Autodesk Inventor part; units mm, degrees
ref_plane "YZ Plane" through (0, 0, 0) normal (1, 0, 0) x (0, 1, 0)
ref_plane "XZ Plane" through (0, 0, 0) normal (0, 1, 0) x (-1, 0, 0)
ref_plane "XY Plane" through (0, 0, 0) normal (0, 0, 1) x (1, 0, 0)
sketch "Sketch1" plane through (0, 0, 0) normal (1, 0, 0) x (0, 1, 0)
  line L0 (50, 50) -> (-50, 50)
  line L1 (-50, 50) -> (-50, -50)
  line L2 (-50, -50) -> (50, -50)
  line L3 (50, -50) -> (50, 50)
  line L4 (50, 50) -> (-50, -50) construction
  line L5 (-50, 50) -> (50, -50) construction
  point P0 (0, 0)
  dimension "d0" = 100
  dimension "d1" = 100
extrude "Extrusion1" add sketch "Sketch1" along normal blind 3
sketch "Sketch2" plane through (3, 0, 0) normal (1, 0, 0) x (0, 0, -1)
  circle A0 centre (-8, -9) radius 1.5
  circle A1 centre (8, -9) radius 1.5
  circle A2 centre (8, 9) radius 1.5
  circle A3 centre (-8, 9) radius 1.5
  ellipse E0 centre (0, 0) end of major axis (13, 14) minor radius 3.6924 (4.9841, 0.0284) -> (0.0262, 5.3386) ccw
  ellipse E1 centre (0, 0) end of major axis (-13, 14) minor radius 3.7302 (0.0262, 5.3386) -> (-4.9841, -0.0284) ccw
  ellipse E2 centre (0, 0) end of major axis (13, 14) minor radius 3.6924 (-4.9841, -0.0284) -> (-0.0262, -5.3386) ccw
  ellipse E3 centre (0, 0) end of major axis (-13, 14) minor radius 3.7302 (-0.0262, -5.3386) -> (4.9841, 0.0284) ccw
  point P0 (0, 9.3923)
extrude "Extrusion2" cut sketch "Sketch2" against normal blind 3 contours A0 | A1 | A2 | A3
sketch "Sketch3" plane through (3, 0, 0) normal (1, 0, 0) x (0, 0, -1)
  circle A0 centre (0, 0) radius 2.2245
extrude "Extrusion3" cut sketch "Sketch3" against normal blind 1
properties part number "marker plate"
Input: part model. Units: mm. Frame: model coordinates. A direction names the side the tool comes from. Coordinates: 2 decimals unless noted, no trailing zeros. Loops run counter-clockwise (first coordinate to the right, second up) from the corner with the lowest first, then second, coordinate; pieces in that order, holes last. Notation, with made-up numbers: (-17.75, 44.5) - (26.25, 44.5) arc R21 cw to (26.25, 73.5) - close; hole circle Ø10 at (28, 89.5). An arc over 180 degrees is marked (long way). Answer in a Markdown table with one row per item. Add a question column.
Item 1: Section query A-A on y = -9. Return the cut outline in (x, z), then the cut area to 3 significant figures.
Item 2: Section query B-B on z = 8. Return the cut outline in (x, y).
Item 3: Line query: line 1 along Y through (x, z) = (1.05, 8); line 2 along Y through (x, z) = (2.55, 0); line 3 along Z through (x, y) = (2.7, -0.5). Output: solid intervals per line, ascending. Write a range as [from, to].
Item 4: Access query for faces 1 (the flat face through (3, -1, 12)), 2 (the cylindrical face through (2.51, 0.67, -2.12)). Directions: +Z, -Z, +X, -X, +Y, -Y. A direction counts if a zero-diameter tool reaches every point of the face in a straight line with its end or side. Return the directions, or none.
Item 5: Mould query, pull axis Y, two halves, no side actions, for faces 3 (the cylindrical face through (1.5, -9.9, 9.2)), 4 (the flat face through (1, 50, -1)), 5 (the flat face through (1, -1, -50)). Classes: released by +Y, released by -Y, zero draft, split by the parting line, or undercut.
Recorded:
| question | item | result |
|---|---|---|
| 1 | outline | (0, -50) - (3, -50) - (3, -9.5) - (0, -9.5) - close; (0, -6.5) - (3, -6.5) - (3, 6.5) - (0, 6.5) - close; (0, 9.5) - (3, 9.5) - (3, 50) - (0, 50) - close |
| 1 | area | 282 mm^2 |
| 2 | outline | (0, -50) - (3, -50) - (3, -10.5) - (0, -10.5) - close; (0, -7.5) - (3, -7.5) - (3, 7.5) - (0, 7.5) - close; (0, 10.5) - (3, 10.5) - (3, 50) - (0, 50) - close |
| 3 | line 1 | [-50, -10.5], [-7.5, 7.5], [10.5, 50] |
| 3 | line 2 | [-50, -2.22], [2.22, 50] |
| 3 | line 3 | [-50, -2.17], [2.17, 50] |
| 4 | face 1 | +Z, -Z, +X, +Y, -Y |
| 4 | face 2 | +X |
| 5 | face 3 | undercut |
| 5 | face 4 | released by +Y |
| 5 | face 5 | zero draft |
